Build history of the part. All positions in model axes, mm. Give positions to 0.01 mm unless a question says otherwise; leave off trailing zeros. Write each loop counter-clockwise with the first axis right and the second up, starting at its lowest first coordinate (ties: lowest second). Pieces come first, ordered by that corner, then holes. Notation, with made-up numbers: (67.25, 2.5) -> (126.25, 2.5) arc R13 cw to (126.25, 27.5) -> close; hole circle Ø11 at (75.25, 14.25). An arc over 180 degrees is marked (long way). Put each result on its own line as item: value.
from build123d import *

# Parameters (mm, degrees)
BOSS_EXTRUDE1_DEPTH  = 0.79375
M4_CLEARANCE_HOLE1_D = 4.8
FILLET1_R            = 2.54


with BuildPart() as part:
    # Sketch1 → Boss-Extrude1 (new, symmetric)
    with BuildSketch(Plane.XY):
        with BuildLine():
            Line((-25.4, 0), (25.4, 0))
            Line((25.4, 0), (12.7, 63.5))
            ThreePointArc((12.7, 63.5), (0, 50.8), (-12.7, 63.5))
            Line((-12.7, 63.5), (-25.4, 0))
        make_face()
    extrude(amount=BOSS_EXTRUDE1_DEPTH, both=True)

    # M4 Clearance Hole1 (through all)
    with Locations(Plane.XY.offset(0.79375)):
        with Locations((17.45, 7.62), (-17.45, 7.62)):
            Hole(M4_CLEARANCE_HOLE1_D / 2)

    # Fillet1
    fillet1_edges = [part.edges().sort_by_distance(p)[0] for p in [
        (12.7, 63.5, 0),
        (25.4, 0, 0),
        (-25.4, 0, 0),
        (-12.7, 63.5, 0),
    ]]
    fillet(fillet1_edges, radius=FILLET1_R)


solid = part.part
1) Slice it at B-B (x = 17.45). Write the cut outline in (y, z), plus the area to 3 significant figures.
Filled sheet:
outline: (0, -0.79) -> (5.22, -0.79) -> (5.22, 0.79) -> (0, 0.79) -> close; (10.02, -0.79) -> (39.75, -0.79) -> (39.75, 0.79) -> (10.02, 0.79) -> close
area: 55.5 mm2
2) Slice it at D-D (y = 27.5). Write the cut outline in (x, z), plus the area to 3 significant figures.
Filled sheet:
outline: (-19.9, -0.79) -> (19.9, -0.79) -> (19.9, 0.79) -> (-19.9, 0.79) -> close
area: 63.2 mm2
3) Slice it at A-A (z = 0). Write the cut outline in (x, y).
Filled sheet:
outline: (-24.79, 3.04) arc R2.54 ccw to (-22.3, 0) -> (22.3, 0) arc R2.54 ccw to (24.79, 3.04) -> (14.48, 54.59) arc R2.54 ccw to (9.99, 55.66) arc R12.7 cw to (-9.99, 55.66) arc R2.54 ccw to (-14.48, 54.59) -> close; hole circle Ø4.8 at (-17.45, 7.62); hole circle Ø4.8 at (17.45, 7.62)
4) Pull direction X, two halves, no side cores. Call faces 1 (the cylindrical face through (24.25, 0.91, 0.01)), 2 (the flat face through (0, 22, -0.794)), 3 (the cylindrical face through (12.619, 56.555, 0.011)), 4 (the cylindrical face through (19.22, 9.24, -0.01)): released by +X, released by -X, zero draft, split by the parting line, or undercut.
Filled sheet:
face 1: released by +X
face 2: zero draft
face 3: undercut
face 4: undercut
5) Wall check: L1, parallel to X at y = 6.5, z = 0.65; L2, parallel to X at y = 8, z = 0.5; L3, parallel to X at y = 53.5, z = 0.65. Give the ranges that are in metal, low to high.
Filled sheet:
L1: -24.1 to -19.57, -15.33 to 15.33, 19.57 to 24.1
L2: -23.8 to -19.82, -15.08 to 15.08, 19.82 to 23.8
L3: -14.7 to -7.83, 7.83 to 14.7
6) Slice it at C-C (y = 7.62). Write the cut outline in (x, z), plus the area to 3 significant figures.
Filled sheet:
outline: (-23.88, -0.79) -> (-19.85, -0.79) -> (-19.85, 0.79) -> (-23.88, 0.79) -> close; (-15.05, -0.79) -> (15.05, -0.79) -> (15.05, 0.79) -> (-15.05, 0.79) -> close; (19.85, -0.79) -> (23.88, -0.79) -> (23.88, 0.79) -> (19.85, 0.79) -> close
area: 60.6 mm2
